from build123d import *

# Parameters (mm, degrees)
BOSS_EXTRUDE1_DEPTH                           = 15.875
BOSS_EXTRUDE2_DEPTH                           = 15.875
CBORE_FOR_1_4_SOCKET_HEAD_CAP_SCREW1_AT_COUNT = 2
CBORE_FOR_1_4_SOCKET_HEAD_CAP_SCREW1_AT_PITCH = 53.975
MOVE_FACE1_BY                                 = 0.127
MOVE_FACE1_2_BY                               = 0.127
MOVE_START                                    = 28.575
MOVE_FACE2_OUTLINE_W                          = 15.875
MOVE_FACE2_OUTLINE_H                          = 73.025
MOVE_FACE2_OUTLINE_R                          = 5.55625
MOVE_FACE2_DEPTH                              = 6.35
MOVE_START_2                                  = 22.225
MOVE_FACE2_2_OUTLINE_R                        = 5.55625
MOVE_FACE2_2_OUTLINE_R_2                      = 3.57124
MOVE_FACE2_2_DEPTH                            = 6.35


with BuildPart() as part:
    # Sketch1 → Boss-Extrude1 (new body)
    with BuildSketch(Plane(origin=(0, 0, 0), x_dir=(0, 0, -1), z_dir=(1, 0, 0))):
        with BuildLine():
            Line((36.5125, 0), (20.6375, 0))
            ThreePointArc((20.6375, 0), (0, -20.6375), (-20.6375, 0))
            Line((-20.6375, 0), (-36.5125, 0))
            Line((-36.5125, 0), (-36.5125, -34.925))
            Line((-36.5125, -34.925), (36.5125, -34.925))
            Line((36.5125, -34.925), (36.5125, 0))
        make_face()
    extrude(amount=BOSS_EXTRUDE1_DEPTH)


with BuildPart() as body_2:
    # Sketch1<3> → Boss-Extrude2 (new body)
    with BuildSketch(Plane(origin=(0, 0, 0), x_dir=(0, 0, -1), z_dir=(1, 0, 0))):
        with BuildLine():
            ThreePointArc((-20.6375, 0), (0, 20.6375), (20.6375, 0))
            Line((20.6375, 0), (36.5125, 0))
            Line((36.5125, 0), (36.5125, 34.925))
            Line((36.5125, 34.925), (-36.5125, 34.925))
            Line((-36.5125, 34.925), (-36.5125, 0))
            Line((-36.5125, 0), (-20.6375, 0))
        make_face()
    extrude(amount=BOSS_EXTRUDE2_DEPTH)


with BuildPart() as cbore_for_1_4_socket_head_cap_screw1_tool:
    # Sketch4 → CBORE for 1/4 Socket Head Cap Screw1 (revolve)
    with BuildSketch(Plane(origin=(7.9375, 34.925, 26.9875), x_dir=(0, 0, 1), z_dir=(1, 0, 0))):
        Polygon((0, 0), (0, 69.85), (3.57124, 69.85), (3.57124, 6.35), (5.55625, 6.35), (5.55625, 0.635), (6.19125, 0), align=None)
    cbore_for_1_4_socket_head_cap_screw1 = revolve(axis=Axis((7.9375, 41.275, 26.9875), (0, -1, 0)))


with BuildPart() as part_1:
    add(part.part)

    # CBORE for 1/4 Socket Head Cap Screw1: cut by cbore_for_1_4_socket_head_cap_screw1_tool
    add(cbore_for_1_4_socket_head_cap_screw1_tool.part, mode=Mode.SUBTRACT)


with BuildPart() as body_2_1:
    add(body_2.part)

    # CBORE for 1/4 Socket Head Cap Screw1: cut by cbore_for_1_4_socket_head_cap_screw1_tool
    add(cbore_for_1_4_socket_head_cap_screw1_tool.part, mode=Mode.SUBTRACT)


with BuildPart() as cbore_for_1_4_socket_head_cap_screw1_at_tool:
    # CBORE for 1/4 Socket Head Cap Screw1 at: CBORE for 1/4 Socket Head Cap Screw1 ×2
    with Locations(*[(0, 0, -i * CBORE_FOR_1_4_SOCKET_HEAD_CAP_SCREW1_AT_PITCH) for i in range(1, CBORE_FOR_1_4_SOCKET_HEAD_CAP_SCREW1_AT_COUNT)]):
        add(cbore_for_1_4_socket_head_cap_screw1)


with BuildPart() as part_2:
    add(part_1.part)

    # CBORE for 1/4 Socket Head Cap Screw1 at: cut by cbore_for_1_4_socket_head_cap_screw1_at_tool
    add(cbore_for_1_4_socket_head_cap_screw1_at_tool.part, mode=Mode.SUBTRACT)

    # Move Face1 2: a curved face moved inward by 0.127
    add(Solid.thicken(part_2.faces().sort_by_distance((7.9375, -20.6375, 0))[0], -MOVE_FACE1_2_BY), mode=Mode.SUBTRACT)

    # Chamfer1
    # the kernel refuses this chamfer: 0.635 mm, written as the material it takes off along each edge
    with BuildSketch(Plane(origin=(0, 0, 0), x_dir=(0, 0.07868977926472538, -0.9968991516895122), z_dir=(0, 0.9968991516895122, 0.07868977926472538))) as chamfer1_piece_1:
        with BuildLine():
            Line((21.417460512, 0.017960512), (20.746539488, -0.652960512))
            Line((20.746539488, -0.652960512), (20.733839488, -0.652960512))
            ThreePointArc((20.733839488, -0.652960512), (20.7518, -0.326480256), (20.7518, 0))
            Line((20.7518, 0), (20.7645, 0.0127))
            ThreePointArc((20.7645, 0.0127), (21.090980256, 0.0127), (21.417460512, 0.030660512))
            Line((21.417460512, 0.030660512), (21.417460512, 0.017960512))
        make_face()
    revolve(axis=Axis((0, 0, 0), (-1, 0, 0)), revolution_arc=189.026516368, mode=Mode.SUBTRACT)
    with BuildSketch(Plane(origin=(-1.610111621, 0, -20.7645), x_dir=(0, 0, -1), z_dir=(1, 0, 0))) as chamfer1_piece_2:
        with BuildLine():
            Line((0.643801601, 0.017692029), (-0.027368853, -0.633849299))
            Line((-0.027368853, -0.633849299), (-0.040063261, -0.633472445))
            ThreePointArc((-0.040063261, -0.633472445), (-0.015119867, -0.316902726), (-0.0127, 0))
            Line((-0.0127, 0), (0, 0.0127))
            ThreePointArc((0, 0.0127), (0.3219008, 0.0127), (0.643801601, 0.030392029))
            Line((0.643801601, 0.030392029), (0.643801601, 0.017692029))
        make_face()
    extrude(amount=19.095223242, mode=Mode.SUBTRACT)
    with BuildSketch(Plane(origin=(-1.610111621, 0, 20.7645), x_dir=(0, -0.9998899044534173, -0.01483842889716635), z_dir=(1, 0, 0))) as chamfer1_piece_3:
        with BuildLine():
            Line((0.634185626, 0.017960512), (-0.027243086, -0.643468199))
            Line((-0.027243086, -0.643468199), (-0.039941687, -0.643279751))
            ThreePointArc((-0.039941687, -0.643279751), (-0.017475104, -0.321676913), (-0.012698602, 0.000188448))
            Line((-0.012698602, 0.000188448), (0.000188448, 0.012698602))
            ThreePointArc((0.000188448, 0.012698602), (0.317092192, 0.010415864), (0.633997178, 0.030659114))
            Line((0.633997178, 0.030659114), (0.634185626, 0.017960512))
        make_face()
    extrude(amount=19.095223242, mode=Mode.SUBTRACT)
    with BuildSketch(Plane(origin=(15.875, 0, 0), x_dir=(0, 0.0786897792647254, -0.9968991516895122), z_dir=(0, 0.9968991516895122, 0.0786897792647254))) as chamfer1_piece_4:
        with BuildLine():
            Line((20.746539488, 0.652960512), (21.417460512, -0.017960512))
            Line((21.417460512, -0.017960512), (21.417460512, -0.030660512))
            ThreePointArc((21.417460512, -0.030660512), (21.090980256, -0.0127), (20.7645, -0.0127))
            Line((20.7645, -0.0127), (20.7518, 0))
            ThreePointArc((20.7518, 0), (20.7518, 0.326480256), (20.733839488, 0.652960512))
            Line((20.733839488, 0.652960512), (20.746539488, 0.652960512))
        make_face()
    revolve(axis=Axis((15.875, 0, 0), (-1, 0, 0)), revolution_arc=189.026516368, mode=Mode.SUBTRACT)


with BuildPart() as body_2_2:
    add(body_2_1.part)

    # CBORE for 1/4 Socket Head Cap Screw1 at: cut by cbore_for_1_4_socket_head_cap_screw1_at_tool
    add(cbore_for_1_4_socket_head_cap_screw1_at_tool.part, mode=Mode.SUBTRACT)

    # Move Face1: a curved face moved inward by 0.127
    add(Solid.thicken(body_2_2.faces().sort_by_distance((7.9375, 20.6375, 0))[0], -MOVE_FACE1_BY), mode=Mode.SUBTRACT)

    # Move Face2: read off the stored shape, not the designer's step
    # Move Face2 outline → Move Face2 (cut)
    with BuildSketch(Plane(origin=(0, 0, 0), x_dir=(1, 0, 0), z_dir=(0, 1, 0)).offset(MOVE_START)):
        with Locations((7.9375, 0)):
            Rectangle(MOVE_FACE2_OUTLINE_W, MOVE_FACE2_OUTLINE_H)
        with Locations((7.9375, -26.9875)):
            Circle(MOVE_FACE2_OUTLINE_R, mode=Mode.SUBTRACT)
        with Locations((7.9375, 26.9875)):
            Circle(MOVE_FACE2_OUTLINE_R, mode=Mode.SUBTRACT)
    extrude(amount=MOVE_FACE2_DEPTH, mode=Mode.SUBTRACT)

    # Move Face2 2 outline → Move Face2 2 (cut)
    # profile 1 of 2: a face of its own
    with BuildSketch(Plane(origin=(0, 0, 0), x_dir=(1, 0, 0), z_dir=(0, 1, 0)).offset(MOVE_START_2)):
        with Locations((7.9375, 26.9875)):
            Circle(MOVE_FACE2_2_OUTLINE_R)
        with Locations((7.9375, 26.9875)):
            Circle(MOVE_FACE2_2_OUTLINE_R_2, mode=Mode.SUBTRACT)
    # profile 2 of 2: a face of its own
    with BuildSketch(Plane(origin=(0, 0, 0), x_dir=(1, 0, 0), z_dir=(0, 1, 0)).offset(MOVE_START_2)):
        with Locations((7.9375, -26.9875)):
            Circle(MOVE_FACE2_2_OUTLINE_R)
        with Locations((7.9375, -26.9875)):
            Circle(MOVE_FACE2_2_OUTLINE_R_2, mode=Mode.SUBTRACT)
    extrude(amount=MOVE_FACE2_2_DEPTH, mode=Mode.SUBTRACT)

    # Move Face2 3: loft between two sections, ruled curve by curve
    move_face2_3_from = [
        Edge.make_three_point_arc((7.9375, 27.94, -21.43125), (13.49375, 27.94, -26.9875), (7.9375, 27.94, -32.54375)),
        Edge.make_three_point_arc((7.9375, 27.94, -32.54375), (2.38125, 27.94, -26.9875), (7.9375, 27.94, -21.43125)),
    ]
    move_face2_3_to = [
        Edge.make_three_point_arc((7.9375, 28.575, -20.79625), (14.12875, 28.575, -26.9875), (7.9375, 28.575, -33.17875)),
        Edge.make_three_point_arc((7.9375, 28.575, -33.17875), (1.74625, 28.575, -26.9875), (7.9375, 28.575, -20.79625)),
    ]
    move_face2_3 = Solid(Shell([*[Face.make_surface_from_curves(move_face2_3_from[k], move_face2_3_to[k]) for k in range(2)], Face(Wire(move_face2_3_from)), Face(Wire(move_face2_3_to))]))
    add(move_face2_3, mode=Mode.SUBTRACT)

    # Move Face2 4: loft between two sections, ruled curve by curve
    move_face2_4_from = [
        Edge.make_three_point_arc((7.9375, 27.94, 32.54375), (13.49375, 27.94, 26.9875), (7.9375, 27.94, 21.43125)),
        Edge.make_three_point_arc((7.9375, 27.94, 21.43125), (2.38125, 27.94, 26.9875), (7.9375, 27.94, 32.54375)),
    ]
    move_face2_4_to = [
        Edge.make_three_point_arc((7.9375, 28.575, 33.17875), (14.12875, 28.575, 26.9875), (7.9375, 28.575, 20.79625)),
        Edge.make_three_point_arc((7.9375, 28.575, 20.79625), (1.74625, 28.575, 26.9875), (7.9375, 28.575, 33.17875)),
    ]
    move_face2_4 = Solid(Shell([*[Face.make_surface_from_curves(move_face2_4_from[k], move_face2_4_to[k]) for k in range(2)], Face(Wire(move_face2_4_from)), Face(Wire(move_face2_4_to))]))
    add(move_face2_4, mode=Mode.SUBTRACT)

    # Chamfer2
    # the kernel refuses this chamfer: 0.635 mm, written as the material it takes off along each edge
    with BuildSketch(Plane(origin=(0, 0, 0), x_dir=(0, -0.0786897792647251, 0.9968991516895122), z_dir=(0, -0.9968991516895122, -0.0786897792647251))) as chamfer2_piece_1:
        with BuildLine():
            Line((21.417460512, 0.017960512), (20.746539488, -0.652960512))
            Line((20.746539488, -0.652960512), (20.733839488, -0.652960512))
            ThreePointArc((20.733839488, -0.652960512), (20.7518, -0.326480256), (20.7518, 0))
            Line((20.7518, 0), (20.7645, 0.0127))
            ThreePointArc((20.7645, 0.0127), (21.090980256, 0.0127), (21.417460512, 0.030660512))
            Line((21.417460512, 0.030660512), (21.417460512, 0.017960512))
        make_face()
    revolve(axis=Axis((0, 0, 0), (-1, 0, 0)), revolution_arc=189.026516368, mode=Mode.SUBTRACT)
    with BuildSketch(Plane(origin=(-1.610111621, 0, 20.7645), x_dir=(0, 0, 1), z_dir=(1, 0, 0))) as chamfer2_piece_2:
        with BuildLine():
            Line((0.643801601, 0.017692029), (-0.027368853, -0.633849299))
            Line((-0.027368853, -0.633849299), (-0.040063261, -0.633472445))
            ThreePointArc((-0.040063261, -0.633472445), (-0.015119867, -0.316902726), (-0.0127, 0))
            Line((-0.0127, 0), (0, 0.0127))
            ThreePointArc((0, 0.0127), (0.3219008, 0.0127), (0.643801601, 0.030392029))
            Line((0.643801601, 0.030392029), (0.643801601, 0.017692029))
        make_face()
    extrude(amount=19.095223242, mode=Mode.SUBTRACT)
    with BuildSketch(Plane(origin=(-1.610111621, 0, -20.7645), x_dir=(0, 0.9998899044534173, 0.014838428897166573), z_dir=(1, 0, 0))) as chamfer2_piece_3:
        with BuildLine():
            Line((0.634185626, 0.017960512), (-0.027243086, -0.643468199))
            Line((-0.027243086, -0.643468199), (-0.039941687, -0.643279751))
            ThreePointArc((-0.039941687, -0.643279751), (-0.017475104, -0.321676913), (-0.012698602, 0.000188448))
            Line((-0.012698602, 0.000188448), (0.000188448, 0.012698602))
            ThreePointArc((0.000188448, 0.012698602), (0.317092192, 0.010415864), (0.633997178, 0.030659114))
            Line((0.633997178, 0.030659114), (0.634185626, 0.017960512))
        make_face()
    extrude(amount=19.095223242, mode=Mode.SUBTRACT)
    with BuildSketch(Plane(origin=(15.875, 0, 0), x_dir=(0, -0.07868977926472513, 0.9968991516895122), z_dir=(0, -0.9968991516895122, -0.07868977926472513))) as chamfer2_piece_4:
        with BuildLine():
            Line((20.746539488, 0.652960512), (21.417460512, -0.017960512))
            Line((21.417460512, -0.017960512), (21.417460512, -0.030660512))
            ThreePointArc((21.417460512, -0.030660512), (21.090980256, -0.0127), (20.7645, -0.0127))
            Line((20.7645, -0.0127), (20.7518, 0))
            ThreePointArc((20.7518, 0), (20.7518, 0.326480256), (20.733839488, 0.652960512))
            Line((20.733839488, 0.652960512), (20.746539488, 0.652960512))
        make_face()
    revolve(axis=Axis((15.875, 0, 0), (-1, 0, 0)), revolution_arc=189.026516368, mode=Mode.SUBTRACT)


solid = body_2_2.part
Build history of the part. All positions in model axes, mm. A direction names the side the tool comes from. Coordinates: 2 decimals unless noted, no trailing zeros. Order: outer loops, then holes, each group sorted by start corner. A loop starts at its lowest first (then second) coordinate and runs counter-clockwise, first axis right, second up. Notation, with made-up numbers: (76, 52) - (130, 52) arc R20 ccw to (130, 75) - close; hole circle Ø10 at (-3, 29). An arc over 180 degrees is marked (long way). Put each result on its own line as item: value.
1. Probe line 1 along Z through (x, y) = (10.5, 5.75); line 2 along Z through (x, y) = (9.5, 19.25); line 3 along Z through (x, y) = (14.5, 2.5). List the from-to ranges inside material, lowest first. Write a range as [from, to].
Answer sheet:
line 1: z = [-36.51, -29.47], [-24.5, -19.95], [19.95, 24.5], [29.47, 36.51]
line 2: z = [-36.51, -30.2], [-23.78, -7.78], [7.78, 23.78], [30.2, 36.51]
line 3: z = [-36.51, -20.61], [20.61, 36.51]
2. Saw through at A-A (y = 2). Give the number of separate pieces and of enclosed holes in the cut face, and give its area (3 significant figures).
Answer sheet:
separate pieces: 2
enclosed holes: 2
area: 422 mm^2
3. Saw through at C-C (y = 26). Write the cut outline in (x, z) (1 decimal).
Answer sheet:
outline: (0, -36.5) - (15.9, -36.5) - (15.9, 36.5) - (0, 36.5) - close; hole circle Ø11.1 at (7.9, -27); hole circle Ø11.1 at (7.9, 27)
4. Drop flat-ended pins along their axis: P1, Ø8, axis at x = 7.94, z = -26.99, coming from the +Y side (3 decimals); P2, Ø6.5, axis at x = 7.94, z = 26.99, coming from the +Y side; P3, Ø5, axis at x = 8.5, z = 5, coming from the -Y side. Give the stop position or say it passes through.
Answer sheet:
P1: stops at y = 22.225
P2: passes through
P3: stops at y = 19.36
5. Saw through at B-B (z = 0). Write the cut outline in (x, y) (1 decimal), and give its area (3 significant figures).
Answer sheet:
outline: (0, 21.4) - (0.6, 20.8) - (15.2, 20.8) - (15.9, 21.4) - (15.9, 28.6) - (0, 28.6) - close
area: 124 mm^2
6. Tool access for faces 1 (the face through (8, 22.225, -23)), 2 (the face through (8, 0, 31)): list every direction of +Z, -Z, +X, -X, +Y, -Y with a clear straight run to the whole face (end or side of a thin tool).
Answer sheet:
face 1: +Y
face 2: +Z, -Z, +X, -X, -Y
